Build history of the part. All positions in model axes, mm. A direction names the side the tool comes from. Give positions to 0.01 mm unless a question says otherwise; leave off trailing zeros. Order: outer loops, then holes, each group sorted by start corner. A loop starts at its lowest first (then second) coordinate and runs counter-clockwise, first axis right, second up. Notation, with made-up numbers: (69.5, 18.5) - (107.5, 18.5) arc R17 cw to (107.5, 50.5) - close; hole circle Ø7 at (43.25, 86.25). An arc over 180 degrees is marked (long way). Use a Markdown table: item, result. Add a question column.
(1) Slice it at B-B (x = 0). Count the separate pieces of the cut face and the enclosed holes in it, then the cut area to 3 significant figures.
(2) Slice it at C-C (y = -29). Write the cut outline in (x, z), then the cut area to 3 significant figures.
(3) Mould opens along Y. For faces 1 (the face through (3.546, 43.372, 1.479)), 2 (the face through (0, -35, -6)), 3 (the face through (-0.047, 54.132, 1.479)), 4 (the face through (-1, -3, -15)) say: +Y half, -Y half, draft (parallel to the pull), parting line (faces both ways), or undercut.
(4) Slice it at A-A (z = -6). Write the cut outline in (x, y), then the cut area to 3 significant figures.
(5) Wall check: line 1 (Y direction, x = 0, z = -10.25); line 2 (Y direction, x = 0, z = 3.65); line 3 (X direction, y = 34.5, z = 3.3). Give the ranges that are in metal, low to high.
(6) Flat gauge pins, fed straight in: pin 1 (1.5 mm diameter, centred on y = -33.5, z = -11, fed in from -X); pin 2 (2.5 mm diameter, centred on y = -32.5, z = -2.5, fed in from +X); pin 3 (2 mm diameter, centred on y = -5, z = -13, fed in from +X). Where does each tip first touch, or does it go through?
(7) Slice it at D-D (y = -4). Write the cut outline in (x, z), then the cut area to 3 significant figures.
(8) Which spindle directions (+Z, -Z, +X, -X, +Y, -Y) get a long thin tool onto all of the face, cutting with end or side? Do faces 5 (the face through (0, -4, 0)), 6 (the face through (7.5, -33, -7)), 7 (the face through (2, -4, -7)), 8 (the face through (-1, -34, -5)), 9 (the face through (7.5, 26, 2)). Say none if no direction does.
from build123d import *

# Parameters (mm, degrees)
EXTRUDE_1_DEPTH     = 4
CUT_EXTRUDE_1_DEPTH = 3
SKETCH_5_R          = 1.25
CUT_EXTRUDE_2_DEPTH = 12.4
SKETCH_6_W          = 17
SKETCH_6_H          = 35
EXTRUDE_2_DEPTH     = 4
SKETCH_7_W          = 13
SKETCH_7_H          = 24
CUT_EXTRUDE_3_DEPTH = 12.1
SKETCH_8_W          = 4
SKETCH_8_H          = 4
SKETCH_8_R          = 1.25
EXTRUDE_3_DEPTH     = 15
EXTRUDE_4_DEPTH     = 5
SKETCH_10_R         = 1.25
CUT_EXTRUDE_4_DEPTH = 35


with BuildPart() as part:
    # 草圖1 → 填料-伸長1 (new body)
    with BuildSketch(Plane.XY):
        with BuildLine():
            Line((7.5, 0), (7.5, 52))
            ThreePointArc((7.5, 52), (0, 59.5), (-7.5, 52))
            Line((-7.5, 52), (-7.5, 0))
            Line((-7.5, 0), (7.5, 0))
        make_face()
    extrude(amount=EXTRUDE_1_DEPTH)

    # 草圖3 → 除料-伸長1 (cut)
    with BuildSketch(Plane.XY):
        with BuildLine():
            ThreePointArc((-2.132795501, 52), (0, 54.132795501), (2.132795501, 52))
            Line((2.132795501, 52), (5, 34.5))
            Line((5, 34.5), (2.114741289, 16.658021353))
            ThreePointArc((2.114741289, 16.658021353), (-0.171540182, 14.864665347), (-2.142213835, 17))
            Line((-2.142213835, 17), (-5, 34.5))
            Line((-5, 34.5), (-2.132795501, 52))
        make_face()
    extrude(amount=CUT_EXTRUDE_1_DEPTH, mode=Mode.SUBTRACT)

    # 草圖5 → 除料-伸長2 (cut)
    with BuildSketch(Plane.XY):
        with Locations((0, 34.5)):
            Circle(SKETCH_5_R)
    extrude(amount=CUT_EXTRUDE_2_DEPTH, mode=Mode.SUBTRACT)

    # 草圖6 → 填料-伸長2 (add)
    with BuildSketch(Plane.XY):
        with Locations((0, -17.5)):
            Rectangle(SKETCH_6_W, SKETCH_6_H)
    extrude(amount=EXTRUDE_2_DEPTH)

    # 草圖7 → 除料-伸長3 (cut)
    with BuildSketch(Plane.XY):
        with Locations((0, -18)):
            Rectangle(SKETCH_7_W, SKETCH_7_H)
    extrude(amount=CUT_EXTRUDE_3_DEPTH, mode=Mode.SUBTRACT)

    # 草圖8 → 填料-伸長3 (add)
    with BuildSketch(Plane.XY):
        with Locations((0, -4)):
            Rectangle(SKETCH_8_W, SKETCH_8_H)
        with Locations((0, -4)):
            Circle(SKETCH_8_R, mode=Mode.SUBTRACT)
    extrude(amount=-EXTRUDE_3_DEPTH)

    # 草圖9 → 填料-伸長4 (add)
    with BuildSketch(Plane(origin=(0, -35, 0), x_dir=(1, 0, 0), z_dir=(0, 1, 0))):
        Polygon((-7.5, 0), (-3, 0), (-3, 5), (3, 5), (3, 0), (7.5, 0), (7.5, 15), (-7.5, 15), align=None)
    extrude(amount=EXTRUDE_4_DEPTH)

    # 草圖10 → 除料-伸長4 (cut)
    with BuildSketch(Plane.XY):
        with Locations((0, -32.5)):
            Circle(SKETCH_10_R)
    extrude(amount=-CUT_EXTRUDE_4_DEPTH, mode=Mode.SUBTRACT)


solid = part.part
Solution:
| question | item | result |
|---|---|---|
| 1 | separate pieces | 5 |
| 1 | enclosed holes | 0 |
| 1 | area | 209 mm2 |
| 2 | outline | (-8.5, 0) - (-6.5, 0) - (-6.5, 4) - (-8.5, 4) - close; (6.5, 0) - (8.5, 0) - (8.5, 4) - (6.5, 4) - close |
| 2 | area | 16.0 mm2 |
| 3 | face 1 | undercut |
| 3 | face 2 | -Y half |
| 3 | face 3 | undercut |
| 3 | face 4 | draft |
| 4 | outline | (-7.5, -35) - (7.5, -35) - (7.5, -30) - (-7.5, -30) - close; (-2, -6) - (2, -6) - (2, -2) - (-2, -2) - close; hole circle Ø2.5 at (0, -32.5); hole circle Ø2.5 at (0, -4) |
| 4 | area | 81.2 mm2 |
| 5 | line 1 | -35 to -33.75, -31.25 to -30, -6 to -5.25, -2.75 to -2 |
| 5 | line 2 | -35 to -30, -6 to 33.25, 35.75 to 59.5 |
| 5 | line 3 | -7.5 to -1.25, 1.25 to 7.5 |
| 6 | pin 1 | x = -7.5 |
| 6 | pin 2 | x = 7.5 |
| 6 | pin 3 | x = 2 |
| 7 | outline | (-8.5, 0) - (-2, 0) - (-2, -15) - (-1.25, -15) - (-1.25, 0) - (1.25, 0) - (1.25, -15) - (2, -15) - (2, 0) - (8.5, 0) - (8.5, 4) - (-8.5, 4) - close |
| 7 | area | 90.5 mm2 |
| 8 | face 5 | -Z |
| 8 | face 6 | -Z, +X, +Y, -Y |
| 8 | face 7 | -Z, +X, +Y |
| 8 | face 8 | -Y |
| 8 | face 9 | +Z, -Z, +X, +Y |
